Answer from the drawing. Dimensions are ordinates in mm from the lowest x, y and z of the part. A direction names the side the tool comes from. Give positions to 0.01 mm unless a question says otherwise; leave off trailing zeros. Order: outer loops, then holes, each group sorted by start corner. A loop starts at its lowest first (then second) coordinate and runs counter-clockwise, first axis right, second up.
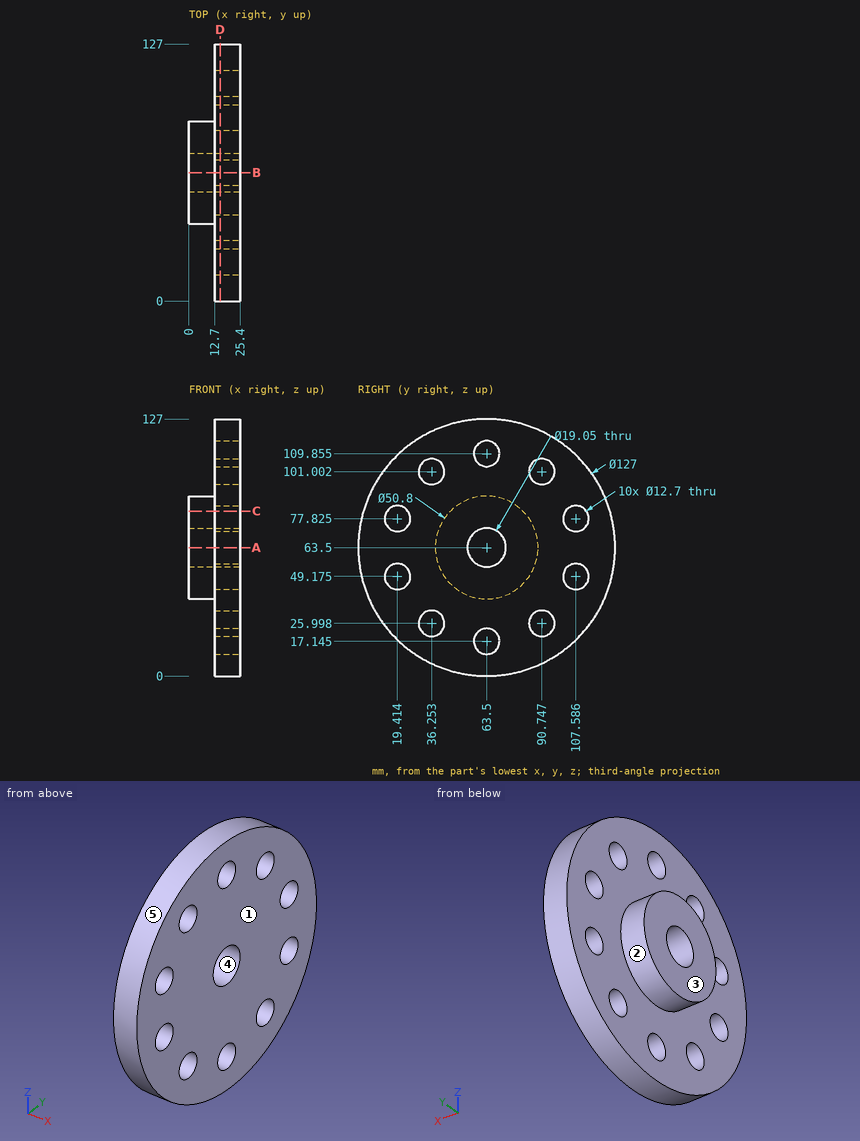
1. Given P1, Ø1, axis at x = 15, y = 102, coming from the -Z side (1 decimal); P2, Ø3, axis at y = 47.5, z = 108, coming from the -X side; P3, Ø11.5, axis at y = 90.75, z = 101, coming from the -X side; P4, Ø10, axis at x = 22, y = 72.5, coming from the +Z side, each flat-ended and moving along its own axis, determine where each tip first touches the part or whether it passes through.
Findings below:
P1: stops at z = 12.6
P2: stops at x = 12.7
P3: passes through
P4: stops at z = 126.87
2. The part is cut by section D-D (x = 15.5). State how many separate pieces and enclosed holes the cut face has, then the cut area to 3 significant figures.
Findings below:
separate pieces: 1
enclosed holes: 11
area: 11,100 mm2
3. The part is cut by section A-A (z = 63.5). Write down the section's boundary in (x, y) (1 decimal).
Findings below:
outline: (0, 38.1) - (12.7, 38.1) - (12.7, 0) - (25.4, 0) - (25.4, 54) - (0, 54) - close; (0, 73) - (25.4, 73) - (25.4, 127) - (12.7, 127) - (12.7, 88.9) - (0, 88.9) - close
4. The part is cut by section C-C (z = 81.5). Write down the section's boundary in (x, y) (1 decimal), then the cut area to 3 significant figures.
Findings below:
outline: (0, 45.6) - (12.7, 45.6) - (12.7, 24.6) - (25.4, 24.6) - (25.4, 102.4) - (12.7, 102.4) - (12.7, 81.4) - (0, 81.4) - close; (12.7, 2.6) - (25.4, 2.6) - (25.4, 14.2) - (12.7, 14.2) - close; (12.7, 112.8) - (25.4, 112.8) - (25.4, 124.4) - (12.7, 124.4) - close
area: 1,740 mm2
5. The mould has two halves that part along Y. Classify the marked faces 3, 4 and 5: pulls with the +Y half, pulls with the -Y half, needs draft (parallel to the pull), parting line crosses it, or undercut.
Findings below:
face 3: needs draft
face 4: undercut
face 5: parting line crosses it
6. Straight lines are drawn through the part: probe 1 along Z at (x, y) = (6.5, 63.5) (1 decimal); probe 2 along Z at (x, y) = (16.75, 112) (1 decimal); probe 3 along Z at (x, y) = (18, 62) (1 decimal). For each, find the intervals that lie inside material, in ascending order.
Findings below:
probe 1: z = 38.1 to 54, 73 to 88.9
probe 2: z = 22.5 to 44.6, 53.7 to 73.3, 82.4 to 104.5
probe 3: z = 0 to 11, 23.3 to 54.1, 72.9 to 103.7, 116 to 127
7. The part is cut by section B-B (y = 63.5). Write down the section's boundary in (x, z) (1 decimal), then the cut area to 3 significant figures.
Findings below:
outline: (0, 38.1) - (12.7, 38.1) - (12.7, 23.5) - (25.4, 23.5) - (25.4, 54) - (0, 54) - close; (0, 73) - (25.4, 73) - (25.4, 103.5) - (12.7, 103.5) - (12.7, 88.9) - (0, 88.9) - close; (12.7, 0) - (25.4, 0) - (25.4, 10.8) - (12.7, 10.8) - close; (12.7, 116.2) - (25.4, 116.2) - (25.4, 127) - (12.7, 127) - close
area: 1,450 mm2
8. Which of the six approach directions +Z, -Z, +X, -X, +Y, -Y give full straight-line access (tool end or side, diameter ignored) to the marked faces 1 and 2?
Findings below:
face 1: +Z, -Z, +X, +Y, -Y
face 2: -X
